For this review, take the finished solid that the model builds, in its own axes (mm). A direction names the side the tool comes from. Coordinates: 2 decimals unless noted, no trailing zeros. Loops run counter-clockwise (first coordinate to the right, second up) from the corner with the lowest first, then second, coordinate; pieces in that order, holes last.
1. Take a section at A-A, the plane z = 241.3. State the section outline as (x, y) points.
2. To check wall thickness, follow probe 1 along Y at (x, z) = (18, 117.5); probe 2 along X at (y, z) = (0.5, 241.3). State the ranges of each line that lie inside material, in increasing order.
3. Take a section at B-B, the plane x = 7. State the section outline as (y, z) points.
4. Take a section at D-D, the plane x = 25.4. Count the separate pieces of the cut face and the enclosed holes in it, then the cut area to 3 significant figures.
5. Machinability: for faces 5 (the face through (25, 1.587, 150)), 6 (the face through (11.234, 0.805, 65.36)), which of the approach directions +Z, -Z, +X, -X, +Y, -Y give a long, thin tool a straight path to every point of the face, cutting with its end or side? Answer none if there is none.
6. Mouldability with a two-part tool opening along Y and no side actions: class faces 1 (the face through (25, 50.8, 150)), 2 (the face through (23, 1, 0)), 3 (the face through (25, 0, 150)), 4 (the face through (0.8, 8.55, 265.87)) as pulls with the +Y half, pulls with the -Y half, needs draft (parallel to the pull), parting line crosses it, or undercut.
```python
from build123d import *

# Parameters (mm, degrees)
SKETCH2_W               = 50.8
SKETCH2_H               = 50.8
SKETCH2_W_2             = 47.625
SKETCH2_H_2             = 47.625
BOSS_EXTRUDE1_DEPTH     = 304.8
SKETCH3_R               = 14.2875
CUT_EXTRUDE1_DEPTH      = 314.152231351
CUT_EXTRUDE2_DEPTH      = 314.152231351
CUT_EXTRUDE2_DEPTH_BACK = 314.152231351
SKETCH4_R               = 2.54


with BuildPart() as part:
    # Sketch2 → Boss-Extrude1 (new body)
    with BuildSketch(Plane.XY):
        with Locations((25.4, 25.4)):
            Rectangle(SKETCH2_W, SKETCH2_H)
        with Locations((25.4, 25.4)):
            Rectangle(SKETCH2_W_2, SKETCH2_H_2, mode=Mode.SUBTRACT)
    extrude(amount=BOSS_EXTRUDE1_DEPTH)

    # Sketch3 → Cut-Extrude1 (cut, through all)
    with BuildSketch(Plane(origin=(0, 50.8, 0), x_dir=(1, 0, 0), z_dir=(0, 1, 0))):
        with Locations(Location((25.4, -241.3, 0), (0, 0, 270))):
            Circle(SKETCH3_R)
        with Locations(Location((25.4, -174.625, 0), (0, 0, 270))):
            Circle(SKETCH3_R)
        with Locations(Location((25.4, -130.175, 0), (0, 0, 90))):
            Circle(SKETCH3_R)
        with Locations(Location((25.4, -63.5, 0), (0, 0, 90))):
            Circle(SKETCH3_R)
    extrude(amount=-CUT_EXTRUDE1_DEPTH, mode=Mode.SUBTRACT)

    # Sketch4 → Cut-Extrude2 (cut, two sides: drawn at the far end of the back side and taken through both)
    with BuildSketch(Plane.ZY.offset(-CUT_EXTRUDE2_DEPTH_BACK)):
        with Locations((9.525, 41.275)):
            Circle(SKETCH4_R)
        with Locations((9.525, 9.525)):
            Circle(SKETCH4_R)
        with Locations((41.275, 41.275)):
            Circle(SKETCH4_R)
        with Locations((41.275, 9.525)):
            Circle(SKETCH4_R)
        with Locations((263.525, 9.525)):
            Circle(SKETCH4_R)
        with Locations((263.525, 41.275)):
            Circle(SKETCH4_R)
        with Locations((295.275, 9.525)):
            Circle(SKETCH4_R)
        with Locations((295.275, 41.275)):
            Circle(SKETCH4_R)
    extrude(amount=CUT_EXTRUDE2_DEPTH + CUT_EXTRUDE2_DEPTH_BACK, mode=Mode.SUBTRACT)


solid = part.part
```
Results list:
1. outline: (0, 0) - (11.11, 0) - (11.11, 1.59) - (1.59, 1.59) - (1.59, 49.21) - (11.11, 49.21) - (11.11, 50.8) - (0, 50.8) - close; (39.69, 0) - (50.8, 0) - (50.8, 50.8) - (39.69, 50.8) - (39.69, 49.21) - (49.21, 49.21) - (49.21, 1.59) - (39.69, 1.59) - close
2. probe 1: y = 0 to 1.59, 49.21 to 50.8
2. probe 2: x = 0 to 11.11, 39.69 to 50.8
3. outline: (0, 0) - (1.59, 0) - (1.59, 304.8) - (0, 304.8) - close; (49.21, 0) - (50.8, 0) - (50.8, 304.8) - (49.21, 304.8) - close
4. separate pieces: 10
4. enclosed holes: 0
4. area: 605 mm2
5. face 5: +Z, -Z
5. face 6: +Y, -Y
6. face 1: pulls with the +Y half
6. face 2: needs draft
6. face 3: pulls with the -Y half
6. face 4: undercut
